from build123d import *

# Parameters (mm, degrees)
SKETCH1_R               = 10
BOSS_EXTRUDE1_DEPTH     = 1
SKETCH2_R               = 10
BOSS_EXTRUDE2_DEPTH     = 4
SKETCH4_R               = 13
BOSS_EXTRUDE3_DEPTH     = 1
CUT_SWEEP1_START        = 4.993438222
CUT_SWEEP1_DEPTH        = 4.55597903
SKETCH9_R               = 1
CUT_EXTRUDE2_DEPTH      = 5
SKETCH10_R              = 2.5
SKETCH10_R_2            = 1
BOSS_EXTRUDE4_DEPTH     = 1
SKETCH11_R              = 13
SKETCH11_R_2            = 10
BOSS_EXTRUDE5_DEPTH     = 1
CUT_EXTRUDE4_DEPTH      = 20.05255902
CUT_EXTRUDE4_DEPTH_BACK = 20.05255902


# Read off the part's stored shape, not the designer's step: Cut-Sweep1
with BuildPart() as part:
    # Sketch1 → Boss-Extrude1 (new body)
    with BuildSketch(Plane(origin=(0, 0, 0), x_dir=(1, 0, 0), z_dir=(0, 1, 0))):
        with Locations(Location((0, 0, 0), (0, 0, 270))):
            Circle(SKETCH1_R)
    extrude(amount=BOSS_EXTRUDE1_DEPTH)

    # Sketch2 → Boss-Extrude2 (add)
    with BuildSketch(Plane(origin=(0, 0, 0), x_dir=(1, 0, 0), z_dir=(0, 1, 0))):
        with Locations(Location((0, 0, 0), (0, 0, 270))):
            Circle(SKETCH2_R)
    extrude(amount=BOSS_EXTRUDE2_DEPTH)

    # Sketch4 → Boss-Extrude3 (add)
    with BuildSketch(Plane(origin=(0, 4, 0), x_dir=(1, 0, 0), z_dir=(0, 1, 0))):
        with Locations(Location((0, 0, 0), (0, 0, 270))):
            Circle(SKETCH4_R)
    extrude(amount=BOSS_EXTRUDE3_DEPTH)

    # Cut-Sweep1 outline → Cut-Sweep1 (cut)
    with BuildSketch(Plane(origin=(0, 0, 0), x_dir=(1, 0, 0), z_dir=(0, 0.6401843996644766, 0.7682212795973786)).offset(CUT_SWEEP1_START)):
        with BuildLine():
            add(Edge.make_bspline(
                [(0, -4.801382997), (1, -4.801382997), (1, -4.161198598), (0, -4.161198598), (-1, -4.161198598), (-1, -4.801382997), (0, -4.801382997)],
                knots=[0, 0, 0, 0, 0.5, 0.5, 0.5, 1, 1, 1, 1], degree=3, weights=[1, 0.333333333, 0.333333333, 1, 0.333333333, 0.333333333, 1]))
        make_face()
    extrude(amount=CUT_SWEEP1_DEPTH, mode=Mode.SUBTRACT)

    # Sketch9 → Cut-Extrude2 (cut)
    with BuildSketch(Plane(origin=(0, 0, 0), x_dir=(1, 0, 0), z_dir=(0, 1, 0))):
        with Locations(Location((0, 0, 0), (0, 0, 270))):
            Circle(SKETCH9_R)
    extrude(amount=CUT_EXTRUDE2_DEPTH, mode=Mode.SUBTRACT)

    # Sketch10 → Boss-Extrude4 (add)
    with BuildSketch(Plane(origin=(0, 0, 0), x_dir=(1, 0, 0), z_dir=(0, 1, 0))):
        Circle(SKETCH10_R)
        with Locations(Location((0, 0, 0), (0, 0, 270))):
            Circle(SKETCH10_R_2, mode=Mode.SUBTRACT)
    extrude(amount=BOSS_EXTRUDE4_DEPTH)

    # Sketch11 → Boss-Extrude5 (add)
    with BuildSketch(Plane(origin=(0, 0, 0), x_dir=(-1, 0, 0), z_dir=(0, -1, 0))):
        with Locations(Location((0, 0, 0), (0, 0, 270))):
            Circle(SKETCH11_R)
        with Locations(Location((0, 0, 0), (0, 0, 90))):
            Circle(SKETCH11_R_2, mode=Mode.SUBTRACT)
    extrude(amount=-BOSS_EXTRUDE5_DEPTH)

    # Sketch12 → Cut-Extrude4 (cut, two sides: drawn at the far end of the back side and taken through both)
    with BuildSketch(Plane(origin=(0, 0, 0), x_dir=(1, 0, 0), z_dir=(0, 1, 0)).offset(-CUT_EXTRUDE4_DEPTH_BACK)):
        with BuildLine():
            Line((-2.233271143, 1.85), (2.233271143, 1.85))
            ThreePointArc((2.233271143, 1.85), (2.9, 0), (2.233271143, -1.85))
            Line((2.233271143, -1.85), (-2.233271143, -1.85))
            ThreePointArc((-2.233271143, -1.85), (-2.9, 0), (-2.233271143, 1.85))
        make_face()
    extrude(amount=CUT_EXTRUDE4_DEPTH + CUT_EXTRUDE4_DEPTH_BACK, mode=Mode.SUBTRACT)


solid = part.part
Build history of the part. All positions in model axes, mm. A direction names the side the tool comes from. Give positions to 0.01 mm unless a question says otherwise; leave off trailing zeros. Order: outer loops, then holes, each group sorted by start corner. A loop starts at its lowest first (then second) coordinate and runs counter-clockwise, first axis right, second up. Notation, with made-up numbers: M -0.5,-18 L 48.5,-18 A19 ccw 48.5,-13 Z; hole C -16,46 d3. An arc over 180 degrees is marked long. Put each result on its own line as item: value.
Item 1: Cut at A-A on z = 0. Write the cut outline in (x, y).
Results are:
outline: M -13,0 L -2.9,0 L -2.9,5 L -13,5 L -13,4 L -10,4 L -10,1 L -13,1 Z; M 2.9,0 L 13,0 L 13,1 L 10,1 L 10,4 L 13,4 L 13,5 L 2.9,5 Z
Item 2: Cut at C-C on x = 3.75. Write the cut outline in (y, z), then the cut area to 3 significant figures.
Results are:
outline: M 0,-12.45 L 1,-12.45 L 1,-9.27 L 4,-9.27 L 4,-12.45 L 5,-12.45 L 5,12.45 L 4,12.45 L 4,9.27 L 1,9.27 L 1,12.45 L 0,12.45 Z
area: 105 mm2
Item 3: Drop flat-ended pins along their axis: pin 1 Ø3 at (y, z) = (1.5, -5) entering from -X; pin 2 Ø3 at (y, z) = (0.5, 4) entering from -X; pin 3 Ø1.5 at (y, z) = (0.5, -5.5) entering from +X. Give the stop position or say it passes through.
Results are:
pin 1: x = -12.5
pin 2: x = -12.76
pin 3: x = 12.1
Item 4: Cut at B-B on y = 3.7. Write the cut outline in (x, z), then the cut area to 3 significant figures.
Results are:
outline: C 0,0 d20; hole M -2.23,-1.85 L 2.23,-1.85 A2.9 ccw 2.23,1.85 L -2.23,1.85 A2.9 ccw Z
area: 294 mm2
Item 5: Pull direction X, two halves, no side cores. Call faces 1 (the face through (7.91, 0.493, -10.316)), 2 (the face through (-8, 4, 7)), 3 (the face through (0, 2, 1.85)): +X half, -X half, draft (parallel to the pull), parting line (faces both ways), or undercut.
Results are:
face 1: parting line
face 2: draft
face 3: undercut
Item 6: Wall check: probe 1 along Y at (x, z) = (-5.5, 10.5); probe 2 along Z at (x, y) = (-2.5, 4.05); probe 3 along X at (y, z) = (0.3, -0.5). Give the ranges that are in metal, low to high.
Results are:
probe 1: 0 to 1, 4 to 5
probe 2: -12.76 to -1.47, 1.47 to 12.76
probe 3: -12.99 to -2.86, 2.86 to 12.99
Item 7: Which spindle directions (+Z, -Z, +X, -X, +Y, -Y) get a long thin tool onto all of the face, cutting with end or side? Do faces 4 (the face through (-2.9, 2.5, 0)), 5 (the face through (-9.76, 2.48, -2.17)), 6 (the face through (0, 0, 3)). Say none if no direction does.
Results are:
face 4: +Y, -Y
face 5: none
face 6: +Z, -Z, +X, -X, -Y
Item 8: Cut at D-D on z = 10.5. Write the cut outline in (x, y).
Results are:
outline: M -7.66,0 L 7.66,0 L 7.66,1 L -7.66,1 Z; M -7.66,4 L 7.66,4 L 7.66,5 L -7.66,5 Z
